Part model, mm, in its own coordinate system. A direction names the side the tool comes from. Round coordinates to 2 decimals unless told otherwise and drop trailing zeros. Loops run counter-clockwise (first coordinate to the right, second up) from the corner with the lowest first, then second, coordinate; pieces in that order, holes last. Notation, with made-up numbers: (32.25, 57.5) -> (67.25, 57.5) arc R18 cw to (67.25, 71.5) -> close; hole circle Ø1 at (62, -26). An arc over 180 degrees is marked (long way). Use a Markdown table: item, result. Add a question column.
Item 1: Two-plate mould, pull along Y, no slides. Class faces 1 (the face through (-8, 18, 0)), 2 (the face through (0, 30, 2.25)), 3 (the face through (6, 34, 1)): pulls with the +Y half, pulls with the -Y half, needs draft (parallel to the pull), parting line crosses it, or undercut.
Item 2: Cut at A-A, the plane x = -1.5. State how many separate pieces and enclosed holes the cut face has, plus the area to 3 significant figures.
Item 3: Cut at C-C, the plane z = 1.5. List the corners of the cut face in (x, y).
Item 4: Cut at B-B, the plane y = 14. List the corners of the cut face in (x, z), plus the area to 4 significant figures.
Item 5: Probe line 1 (X direction, y = 30, z = 1.75); line 2 (Y direction, x = 2.25, z = 1.5); line 3 (X direction, y = 27, z = 2). List the from-to ranges inside material, lowest first. Write a range as [from, to].
Item 6: Flat gauge pins, fed straight in: pin 1 (1.6 mm diameter, centred on x = 0, y = 29.5, fed in from -Z); pin 2 (0.8 mm diameter, centred on x = -5.5, z = 1.5, fed in from +Y); pin 3 (1.2 mm diameter, centred on x = 6, z = 1, fed in from -Y). Where does each tip first touch, or does it go through?
Item 7: Which spindle directions (+Z, -Z, +X, -X, +Y, -Y) get a long thin tool onto all of the face, cutting with end or side? Do faces 4 (the face through (-6, 22, 1)), 5 (the face through (0, 30, 0.25)), 6 (the face through (5, 5, 1)), 7 (the face through (-1, 13, 2.5)). Say none if no direction does.
```python
from build123d import *

# Parameters (mm, degrees)
F0_W     = 6
F0_H     = 2
F1_DEPTH = 2.5
F2_W     = 8
F2_H     = 4
F3_DEPTH = 4.5
F4_SIZE2 = 3.99999
F4_SIZE  = 2.99999
F5_SIZE2 = 1
F5_SIZE  = 5
F6_W     = 2
F6_H     = 3
F7_DEPTH = 0.25
F8_W     = 2
F8_H     = 3
F9_DEPTH = 0.25


# Not quite as in the source:
# - a fillet or chamfer is up to 0.001 mm smaller than in the source, because OpenCascade refuses the exact size


with BuildPart() as f1:
    # F0 (on Top) → F1 (new body)
    with BuildSketch(Plane.XY):
        Polygon((-5, 11), (-5, 0), (5, 0), (5, 11), (8.75, 11), (8.75, 34), (4, 34), (4, 40), (-4, 40), (-4, 34), (-8.75, 34), (-8.75, 11), align=None)
        with Locations((0, 3)):
            Rectangle(F0_W, F0_H, mode=Mode.SUBTRACT)
        Polygon((-6, 13.5), (-6, 31.5), (-1, 31.5), (-1, 28.5), (1, 28.5), (1, 31.5), (6, 31.5), (6, 13.5), align=None, mode=Mode.SUBTRACT)
    extrude(amount=F1_DEPTH)

    # F2 (on face) → F3 (join)
    with BuildSketch(Plane.XY.offset(2.5)):
        with Locations((0, 38)):
            Rectangle(F2_W, F2_H)
    extrude(amount=F3_DEPTH)

    # F4 (size 3 and 4 in the source; OpenCascade refuses exactly that, so slightly less here)
    f4_edges = [f1.edges().sort_by_distance(p)[0] for p in [
        (0, 40, 7),
    ]]
    f4_side = f1.faces().sort_by_distance((0, 40, 3.5))[0]
    chamfer(f4_edges, length=F4_SIZE, length2=F4_SIZE2, reference=f4_side)

    # F5
    f5_edges = [f1.edges().sort_by_distance(p)[0] for p in [
        (0, 40, 0),
    ]]
    f5_side = f1.faces().sort_by_distance((-4.563394, 5.5, 0))[0]
    chamfer(f5_edges, length=F5_SIZE, length2=F5_SIZE2, reference=f5_side)

    # F6 (on face) → F7 (cut)
    with BuildSketch(Plane.XY.offset(2.5)):
        with Locations((0, 30)):
            Rectangle(F6_W, F6_H)
    extrude(amount=-F7_DEPTH, mode=Mode.SUBTRACT)

    # F8 (on face) → F9 (cut)
    with BuildSketch(Plane(origin=(0, 0, 0), x_dir=(1, 0, 0), z_dir=(0, 0, -1))):
        with Locations((0, -30)):
            Rectangle(F8_W, F8_H)
    extrude(amount=-F9_DEPTH, mode=Mode.SUBTRACT)


solid = f1.part
```
A:
| question | item | result |
|---|---|---|
| 1 | face 1 | needs draft |
| 1 | face 2 | undercut |
| 1 | face 3 | pulls with the +Y half |
| 2 | separate pieces | 3 |
| 2 | enclosed holes | 0 |
| 2 | area | 59.5 mm^2 |
| 3 | outline | (-8.75, 11) -> (-5, 11) -> (-5, 0) -> (5, 0) -> (5, 11) -> (8.75, 11) -> (8.75, 34) -> (4, 34) -> (4, 40) -> (-4, 40) -> (-4, 34) -> (-8.75, 34) -> close; hole (-6, 13.5) -> (6, 13.5) -> (6, 31.5) -> (1, 31.5) -> (1, 28.5) -> (-1, 28.5) -> (-1, 31.5) -> (-6, 31.5) -> close; hole (-3, 2) -> (3, 2) -> (3, 4) -> (-3, 4) -> close |
| 4 | outline | (-8.75, 0) -> (-6, 0) -> (-6, 2.5) -> (-8.75, 2.5) -> close; (6, 0) -> (8.75, 0) -> (8.75, 2.5) -> (6, 2.5) -> close |
| 4 | area | 13.75 mm^2 |
| 5 | line 1 | x = [-8.75, -6], [-1, 1], [6, 8.75] |
| 5 | line 2 | y = [0, 2], [4, 13.5], [31.5, 40] |
| 5 | line 3 | x = [-8.75, -6], [6, 8.75] |
| 6 | pin 1 | stops at z = 0.25 |
| 6 | pin 2 | stops at y = 34 |
| 6 | pin 3 | stops at y = 11 |
| 7 | face 4 | +Z, -Z |
| 7 | face 5 | -Z |
| 7 | face 6 | +Z, -Z, +X, -Y |
| 7 | face 7 | +Z, +X, -X, -Y |
